Autodesk Inventor part; units mm, degrees
ref_plane "Work Plane3" through (-12, 0, 1000) normal (0, -0.9972, -0.0752) x (1, 0, 0)
ref_plane "YZ Plane" through (0, 0, 0) normal (1, 0, 0) x (0, 1, 0)
ref_plane "XZ Plane" through (0, 0, 0) normal (0, 1, 0) x (-1, 0, 0)
sketch "Sketch1" plane through (0, 0, 0) normal (0, 1, 0) x (-1, 0, 0)
  line L0 (-12, 14) -> (12, 14) construction
  line L1 (14, 12) -> (14, -12) construction
  line L2 (12, -14) -> (-12, -14) construction
  line L3 (-14, -12) -> (-14, 12) construction
  line L4 (-14, 14) -> (14, -14) construction
  line L5 (14, 14) -> (-14, -14) construction
  arc A0 (14, 12) -> (12, 14) centre (12, 12) ccw construction
  arc A1 (12, -14) -> (14, -12) centre (12, -12) ccw construction
  arc A2 (-14, -12) -> (-12, -14) centre (-12, -12) ccw construction
  arc A3 (-12, 14) -> (-14, 12) centre (-12, 12) ccw construction
  line L6 (-12, -15) -> (12, -15)
  arc A4 (12, -15) -> (15, -12) centre (12, -12) ccw
  line L7 (15, -12) -> (15, 12)
  arc A5 (15, 12) -> (12, 15) centre (12, 12) ccw
  line L8 (12, 15) -> (-12, 15)
  arc A6 (-12, 15) -> (-15, 12) centre (-12, 12) ccw
  line L9 (-15, 12) -> (-15, -12)
  arc A7 (-15, -12) -> (-12, -15) centre (-12, -12) ccw
  line L10 (13, -12) -> (13, 12)
  arc A8 (13, 12) -> (12, 13) centre (12, 12) ccw
  line L11 (12, 13) -> (-12, 13)
  arc A9 (-12, 13) -> (-13, 12) centre (-12, 12) ccw
  line L12 (-13, 12) -> (-13, -12)
  arc A10 (-13, -12) -> (-12, -13) centre (-12, -12) ccw
  line L13 (-12, -13) -> (12, -13)
  arc A11 (12, -13) -> (13, -12) centre (12, -12) ccw
  point P0 (0, 0)
  point P1 (0, 0)
  point P2 (0, 0)
  dimension "d10" = 2
  dimension "depth" = 30
  dimension "width" = 30
  dimension "thickness" = 2
sketch "Sketch3" plane through (0, 0, 0) normal (1, 0, 0) x (0, 1, 0)
  line L0 (0, 0) -> (0, 2000) construction
  arc A0 (0, 0) -> (150, 11.314) centre (0, 1000) ccw
  line L1 (0, -403.3894) -> (0, 2400.5649)
  line L2 (-30.3433, 0) -> (182.0598, 0)
  line L3 (0, 1000) -> (151.7165, 0) construction
  dimension "d30" = 2000
  dimension "d31" = 1000
  dimension "d61" = 150
sweep "Sweep1" add profiles "Sketch1" path "Sketch3" path curves A0
ref_plane "Work Plane3" through (-12, 0, 1000) normal (0, -0.9972, -0.0752) x (1, 0, 0)
sketch "Sketch5" plane through (-15, 0, 1000) normal (-1, 0, 0) x (0, 0.9972, 0.0752)
  arc A0 (75.213, 997.1675) -> (-75.213, 997.1675) centre (0, 0) ccw construction
  line L0 (0, 0) -> (0, 1000) construction
  point P0 (-50, 998.7492)
  point P1 (50, 998.7492)
  dimension "d64" = 100
hole "Hole3" at (-15, 124.9773, 7.8404) at (-15, 25.2606, 0.3191) direction (1, 0, 0) diameter 8 depth 40 tip angle 118
equation "\"d10\" = thickness"
equation "\"d31\" = 0.5 * d30"
properties part number "podest duzy profil 7" material "Steel"
Work out the finished part from the listing and answer in its coordinate system (mm). A direction names the side the tool comes from. Round coordinates to 2 decimals unless told otherwise and drop trailing zeros. Loops run counter-clockwise (first coordinate to the right, second up) from the corner with the lowest first, then second, coordinate; pieces in that order, holes last. Notation, with made-up numbers: M 57,67.25 L 66,67.25 A21 ccw 66,105.25 Z; hole C -31.5,18.25 d1. An arc over 180 degrees is marked long. Use CSV: the item, a comma, the result in double quotes.
Q1. A tool of negligible diameter and unlimited length cuts with its end or side. For faces 1 (the cylindrical face through (14.01, 121.01, 7.32)), 2 (the flat face through (13, 74, 4)), 3 (the cylindrical face through (0.17, 75.13, -10.21)), 4 (the cylindrical face through (-0.168, 75.273, 15.874)), from which of +Z, -Z, +X, -X, +Y, -Y can it reach the whole face along a straight path? Write none if from no direction.
Determined:
face 1,"+X, -X"
face 2,"none"
face 3,"-Y"
face 4,"+Y"
Q2. Consider L1, parallel to X at y = 40, z = 6; L2, parallel to Z at x = -2.75, y = 133; L3, parallel to Z at x = -8, y = 96.5. Determine where each line is inside the solid, lowest interval first.
Determined:
L1,"-15 to -13, 13 to 15"
L2,"-6.25 to -4.23, 22 to 24.02"
L3,"-10.4 to -8.39, 17.73 to 19.74"
Q3. Section A-A, the plane x = -8.75 is taken. Determine the outline of the cut face in (y, z).
Determined:
outline,"M 0,-15 A1015 ccw 152.25,-3.52 L 151.95,-1.54 A1013 cw 0,-13 Z; M 0,13 A987 ccw 148.05,24.17 L 147.75,26.14 A985 cw 0,15 Z"
Q4. The mould has two halves that part along Z. Classify faces 5 (the flat face through (-13, 74, 4)), 6 (the flat face through (15, 74, 4)), 7 (the cylindrical face through (-0.168, 77.408, -12.044)): pulls with the +Z half, pulls with the -Z half, needs draft (parallel to the pull), parting line crosses it, or undercut.
Determined:
face 5,"undercut"
face 6,"needs draft"
face 7,"pulls with the -Z half"
Q5. Each of these flat-tipped pins is pushed along its axis until it touches: pin 1 (12 mm diameter, centred on x = -7.5, y = 83, fed in from +Z); pin 2 (8 mm diameter, centred on x = 4.5, z = 4, fed in from +Y); pin 3 (12 mm diameter, centred on x = 6, y = 84.5, fed in from -Z); pin 4 (10 mm diameter, centred on x = -10, y = 90.5, fed in from -Z). Where does it stop, or does it pass through?
Determined:
pin 1,"z = 19.03"
pin 2,"through"
pin 3,"z = -11.96"
pin 4,"z = -11.39"
Q6. Section B-B, the plane z = 2 is taken. Determine the outline of the cut face in (x, y).
Determined:
outline,"M -15,0 L -13,0 L -13,21.63 L -15,21.63 Z; M -15,28.89 L -13,28.89 L -13,151.41 L -15,151.41 Z; M 13,0 L 15,0 L 15,21.63 L 13,21.63 Z; M 13,28.89 L 15,28.89 L 15,151.41 L 13,151.41 Z"
